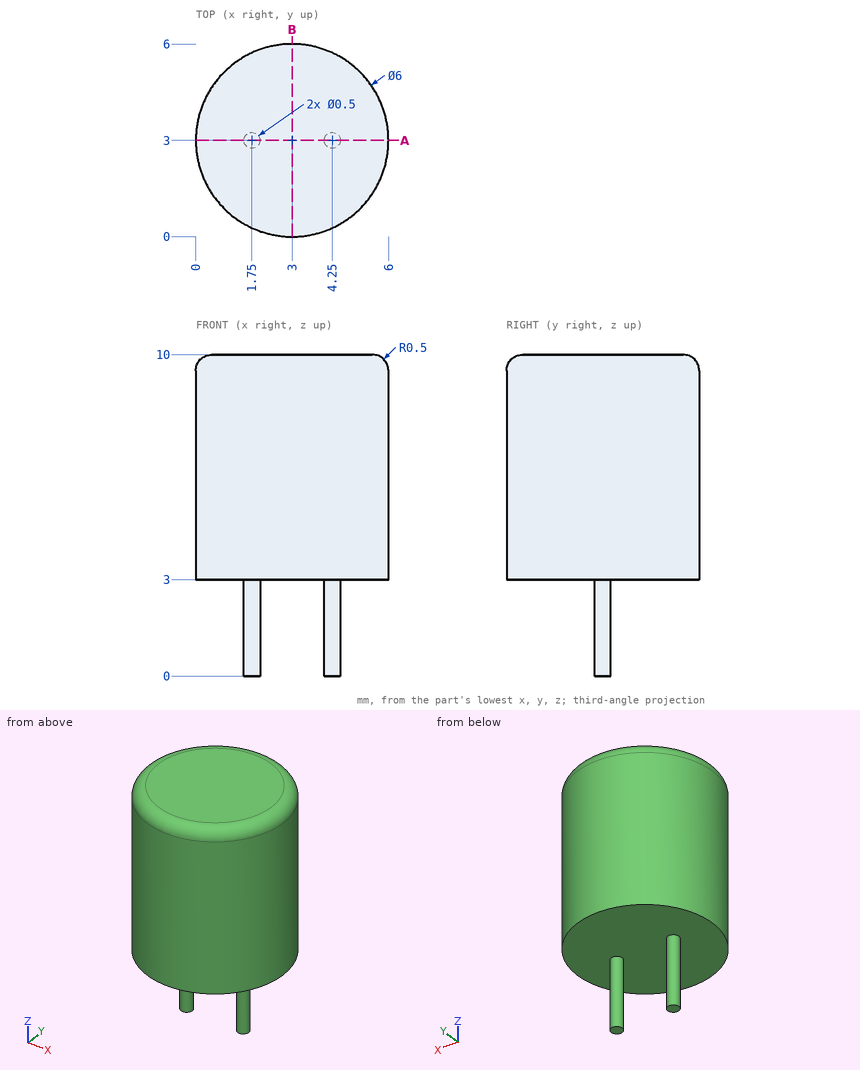
Study the drawing (mm; zero at the part's minimum x, y, z) and answer. Round coordinates to 2 decimals unless told otherwise and drop trailing zeros. Order: outer loops, then holes, each group sorted by start corner. A loop starts at its lowest first (then second) coordinate and runs counter-clockwise, first axis right, second up. Notation, with made-up numbers: (60, -13.75) - (76, -13.75) arc R15 ccw to (76, -2.75) - close; hole circle Ø10 at (87, -32.75). An arc over 180 degrees is marked (long way). Use one line per item in the form item = value. Start each with the question number.
(1) Find the intervals of material crossed by line 1 along Z through (x, y) = (2.4, 1.9); line 2 along X through (y, z) = (5.6, 3.75); line 3 along X through (y, z) = (1.1, 9.5), in increasing order. Write a range as from..to.
(2) Flat-ended cylindrical pins translate along their axes: pin 1 Ø1 at (x, y) = (0.5, 4.5) entering from -Z; pin 2 Ø2 at (y, z) = (1, 8.5) entering from -X. Find the tip coordinate at first contact, or state that the pin passes through.
(3) The part is cut by section A-A (y = 3). Give the vertices of the cut face in (x, z), then the cut area to 3 significant figures.
(4) The part is cut by section B-B (x = 3). Give the vertices of the cut face in (y, z), then the cut area to 3 significant figures.
Checked values:
q1.line_1 = 3..10
q1.line_2 = 1.5..4.5
q1.line_3 = 0.68..5.32
q2.pin_1 = 3
q2.pin_2 = 0.17
q3.outline = (0, 3) - (1.5, 3) - (1.5, 0) - (2, 0) - (2, 3) - (4, 3) - (4, 0) - (4.5, 0) - (4.5, 3) - (6, 3) - (6, 9.5) arc R0.5 ccw to (5.5, 10) - (0.5, 10) arc R0.5 ccw to (0, 9.5) - close
q3.area = 44.9 mm^2
q4.outline = (0, 3) - (6, 3) - (6, 9.5) arc R0.5 ccw to (5.5, 10) - (0.5, 10) arc R0.5 ccw to (0, 9.5) - close
q4.area = 41.9 mm^2
